Verification items for the finished model (mm, model axes). A direction names the side the tool comes from. Coordinates: 2 decimals unless noted, no trailing zeros. Order: outer loops, then holes, each group sorted by start corner. A loop starts at its lowest first (then second) coordinate and runs counter-clockwise, first axis right, second up. Notation, with made-up numbers: (34, 34) -> (56, 34) arc R10 ccw to (56, 53) -> close; hole circle Ø9 at (23, 27.5). An arc over 180 degrees is marked (long way). Write item = value, one per line. Start each with the question number.
1. Cross-section at D-D on y = -128. Record the cut outline in (x, z).
2. Cross-section at A-A on x = 136.5. Record the cut outline in (y, z), plus the area to 3 significant figures.
3. Go/stop test with flat-tipped pins: P1, Ø3, axis at x = 239, z = 76, coming from the -Y side; P2, Ø7.5, axis at x = 230, y = -60.5, coming from the +Z side; P3, Ø7.5, axis at x = 228.5, y = -44, coming from the -Z side. Record where each tip stops, or that it passes through.
4. Set-up check for faces 1 (the flat face through (233, 44.94, 78)), 2 (the flat face through (233, -49, 82.568)), 3 (the flat face through (196.715, -47, 75)): record each of +Z, -Z, +X, -X, +Y, -Y from which the full face is reachable in a straight line by a thin tool's end or side.
5. Cross-section at C-C on y = -2.5. Record the cut outline in (x, z), plus the area to 3 significant figures.
6. Cross-section at B-B on z = 58. Record the cut outline in (x, y).
7. Release check for a two-part mould opening along Y. For faces 4 (the flat face through (81, 29.837, 75)), 5 (the flat face through (82, 51.473, 75)), 6 (the flat face through (233, -49, 73.297)) record: +Y half, -Y half, draft (parallel to the pull), parting line (faces both ways), or undercut.
8. Thickness scan on line 1 along X through (y, z) = (-6, 87); line 2 along Y through (x, z) = (75, 88.5); line 3 along X through (y, z) = (-135, 27). Record the ranges inside material, lowest first. Write a range as from..to.
from build123d import *

# Parameters (mm, degrees)
F0_W     = 272.797018
F0_H     = 198.48334
F0_W_2   = 227.64441
F0_H_2   = 152.390061
F1_DEPTH = 151.892
F2_W     = 184.755966
F2_H     = 9.270906
F3_DEPTH = 25.4


with BuildPart() as f1:
    # F0 (on Top) → F1 (new body)
    with BuildSketch(Plane.XY):
        with Locations((83.833322, -47.768671)):
            Rectangle(F0_W, F0_H)
        with Locations((82.892643, -46.357654)):
            Rectangle(F0_W_2, F0_H_2, mode=Mode.SUBTRACT)
    extrude(amount=F1_DEPTH)

    # F2 (on face) → F3 (join)
    with BuildSketch(Plane.YZ.offset(220.231831)):
        with Locations((-47.437571, 77.932626)):
            Rectangle(F2_W, F2_H)
    extrude(amount=F3_DEPTH)


solid = f1.part
Worked out:
q1.outline = (-52.57, 0) -> (220.23, 0) -> (220.23, 73.3) -> (245.63, 73.3) -> (245.63, 82.57) -> (220.23, 82.57) -> (220.23, 151.89) -> (-52.57, 151.89) -> close
q2.outline = (-147.01, 0) -> (-122.55, 0) -> (-122.55, 151.89) -> (-147.01, 151.89) -> close; (29.84, 0) -> (51.47, 0) -> (51.47, 151.89) -> (29.84, 151.89) -> close
q2.area = 7,000 mm²
q3.P1 = -139.82
q3.P2 = 82.57
q3.P3 = 73.3
q4.face_1 = +Z, -Z, +X, +Y
q4.face_2 = +Z, +X, +Y, -Y
q4.face_3 = +Z, -Z
q5.outline = (-52.57, 0) -> (-30.93, 0) -> (-30.93, 151.89) -> (-52.57, 151.89) -> close; (196.71, 0) -> (220.23, 0) -> (220.23, 73.3) -> (245.63, 73.3) -> (245.63, 82.57) -> (220.23, 82.57) -> (220.23, 151.89) -> (196.71, 151.89) -> close
q5.area = 7,090 mm²
q6.outline = (-52.57, -147.01) -> (220.23, -147.01) -> (220.23, 51.47) -> (-52.57, 51.47) -> close; hole (-30.93, -122.55) -> (196.71, -122.55) -> (196.71, 29.84) -> (-30.93, 29.84) -> close
q7.face_4 = undercut
q7.face_5 = +Y half
q7.face_6 = draft
q8.line_1 = -52.57..-30.93, 196.71..220.23
q8.line_2 = -147.01..-122.55, 29.84..51.47
q8.line_3 = -52.57..220.23
